Here's how the part is built. I have some questions about the finished solid (model axes, mm). A direction names the side the tool comes from. Round coordinates to 2 decimals unless told otherwise and drop trailing zeros. Loops run counter-clockwise (first coordinate to the right, second up) from the corner with the lowest first, then second, coordinate; pieces in that order, holes last. Notation, with made-up numbers: (33, 4.5) -> (90, 4.5) arc R15 ccw to (90, 22.5) -> close; hole circle Ø6 at (44.25, 57). An arc over 180 degrees is marked (long way). Use one line per item in the form item = value. Start each with the question number.
Item 1: If we section it at C-C (x = 0.5): Write out the boundary of the cut face in (y, z) (3 decimals), then the cut area to 3 significant figures.
Item 2: If I drill on L1, parallel to Z at x = -20, y = 0.85 (3 decimals); L2, parallel to X at y = 0.2, z = 5; L3, parallel to Z at x = 27.5, y = 0.6, over which ranges is the centre line in solid material (lowest first)? Write a range as [from, to].
Item 3: I'm going to push flat-ended pins straight in: pin 1 Ø1.6 at (x, y) = (2.5, 1.5) entering from -Z; pin 2 Ø2.5 at (x, z) = (20, 4.76) entering from -Y; pin 3 Ø1.5 at (y, z) = (0.5, 13) entering from -X; pin 4 Ø1.5 at (x, y) = (25.5, 2.5) entering from -Z. Where does each tip first touch, or does it pass through?
Item 4: If we section it at A-A (z = 13.75): Write out the boundary of the cut face in (x, y) (3 decimals), then the cut area to 3 significant figures.
Item 5: If we section it at B-B (y = 2.2): State how many separate pieces and enclosed holes the cut face has, then the cut area to 3 significant figures.
Item 6: For faces 5 (the face through (28.26, 1.61, 0.09)), 6 (the face through (14.097, 1.61, -0.154)), 7 (the face through (26.891, 1.61, -1.808)), 8 (the face through (21.4, 1.61, 14.14)), which set-ups out of +Z, -Z, +X, -X, +Y, -Y let a thin tool reach every point of the face, with its end or its side?
Item 7: Thinking about a two-plate mould opening in Z: for faces 1 (the face through (21.55, 1.61, -4.63)), 2 (the face through (25.12, 1.57, 10.53)), 3 (the face through (29.404, 1.61, 6.003)), 4 (the face through (26.903, 1.565, 8.178)), which applies, released by +Z, released by -Z, zero draft, split by the parting line, or undercut?
```python
from build123d import *

# Parameters (mm, degrees)
CROQUIS1_R              = 1.5875
SALIENTE_EXTRUIR1_DEPTH = 3.175
CROQUIS2_R              = 7.5
CROQUIS2_R_2            = 1.5875
SALIENTE_EXTRUIR2_DEPTH = 3.175
SALIENTE_EXTRUIR3_DEPTH = 3.175
CORTAR_EXTRUIR1_DEPTH   = 10
REDONDEO3_R             = 1
MATRIZC2_COUNT          = 7
MATRIZC2_ANGLE          = 222
REDONDEO3_OF_MATRIZC2_R = 1
REDONDEO4_R             = 2


with BuildPart() as part:
    # Croquis1 → Saliente-Extruir1 (new body)
    with BuildSketch(Plane(origin=(0, 0, 0), x_dir=(1, 0, 0), z_dir=(0, 1, 0))):
        with BuildLine():
            Line((-20, 0), (20, 0))
            ThreePointArc((20, 0), (24.7625, -4.7625), (20, -9.525))
            Line((20, -9.525), (-20, -9.525))
            ThreePointArc((-20, -9.525), (-24.7625, -4.7625), (-20, 0))
        make_face()
        with Locations((-20, -4.7625)):
            Circle(CROQUIS1_R, mode=Mode.SUBTRACT)
        with Locations((20, -4.7625)):
            Circle(CROQUIS1_R, mode=Mode.SUBTRACT)
    extrude(amount=SALIENTE_EXTRUIR1_DEPTH)

    # Croquis2 → Saliente-Extruir2 (add)
    with BuildSketch(Plane(origin=(0, 3.175, 0), x_dir=(1, 0, 0), z_dir=(0, 1, 0))):
        with Locations((20, -4.7625)):
            Circle(CROQUIS2_R)
        with Locations((20, -4.7625)):
            Circle(CROQUIS2_R_2, mode=Mode.SUBTRACT)
    extrude(amount=-SALIENTE_EXTRUIR2_DEPTH)

    # Croquis8 → Saliente-Extruir3 (add)
    with BuildSketch(Plane(origin=(0, 3.175, 0), x_dir=(1, 0, 0), z_dir=(0, 1, 0))):
        with BuildLine():
            Line((14.926688775, 5.835802374), (16.184441281, 1.694396442))
            ThreePointArc((16.184441281, 1.694396442), (17.363636492, 2.258866495), (18.622936274, 2.60999588))
            Line((18.622936274, 2.60999588), (16.844139666, 6.555761596))
            ThreePointArc((16.844139666, 6.555761596), (15.869697171, 6.237640842), (14.926688775, 5.835802374))
        make_face()
    saliente_extruir3 = extrude(amount=-SALIENTE_EXTRUIR3_DEPTH)

    # Croquis9 → Cortar-Extruir1 (cut)
    with BuildSketch(Plane(origin=(0, 3.175, 0), x_dir=(1, 0, 0), z_dir=(0, 1, 0))):
        with BuildLine():
            ThreePointArc((16.844139666, 6.555761596), (16.353447772, 6.407332445), (15.869697296, 6.237640889))
            ThreePointArc((15.869697296, 6.237640889), (16.670669085, 6.223682337), (17.245417982, 5.665637219))
            Line((17.245417982, 5.665637219), (16.844139666, 6.555761596))
        make_face()
        with BuildLine():
            ThreePointArc((15.869697296, 6.237640889), (15.393808961, 6.047009892), (14.926688775, 5.835802374))
            Line((14.926688775, 5.835802374), (15.210424872, 4.901543567))
            ThreePointArc((15.210424872, 4.901543567), (15.275853116, 5.699960746), (15.869697296, 6.237640889))
        make_face()
    cortar_extruir1 = extrude(amount=-CORTAR_EXTRUIR1_DEPTH, mode=Mode.SUBTRACT)

    # Redondeo3
    redondeo3_edges = [part.edges().sort_by_distance(p)[0] for p in [
        (18.622936274, 1.5875, -2.60999588),
        (16.184441281, 1.5875, -1.694396442),
    ]]
    fillet(redondeo3_edges, radius=REDONDEO3_R)

    # MatrizC2: Saliente-Extruir3, Cortar-Extruir1 ×7 about axis
    matrizc2_axis = Axis((20, 0, 4.7625), (0, -1, 0))
    for i in range(1, MATRIZC2_COUNT):
        add(saliente_extruir3.rotate(matrizc2_axis, i * MATRIZC2_ANGLE / (MATRIZC2_COUNT - 1)))
        add(cortar_extruir1.rotate(matrizc2_axis, i * MATRIZC2_ANGLE / (MATRIZC2_COUNT - 1)), mode=Mode.SUBTRACT)

    # Redondeo3 of MatrizC2
    redondeo3_of_matrizc2_edges = [part.edges().sort_by_distance(p)[0] for p in [
        (23.337106788, 1.5875, -1.954174645),
        (20.838616598, 1.5875, -2.690467342),
        (26.707327688, 1.5875, 1.406646118),
        (25.155056708, 1.5875, -0.685012307),
        (27.376313351, 1.5875, 6.118966491),
        (27.395406089, 1.5875, 3.514313802),
        (25.074643863, 1.5875, 10.284998498),
        (26.657411119, 1.5875, 8.216320666),
        (20.729268228, 1.5875, 12.226960319),
        (23.238283761, 1.5875, 11.527373856),
        (16.090195144, 1.5875, 11.16276765),
        (18.515005687, 1.5875, 12.114016299),
    ]]
    fillet(redondeo3_of_matrizc2_edges, radius=REDONDEO3_OF_MATRIZC2_R)

    # Redondeo4
    redondeo4_edges = [part.edges().sort_by_distance(p)[0] for p in [
        (14.206158981, 1.5875, 0),
        (14.206158981, 1.5875, 9.525),
    ]]
    fillet(redondeo4_edges, radius=REDONDEO4_R)


solid = part.part
```
Values found:
q1.outline = (0, 0) -> (3.175, 0) -> (3.175, 9.525) -> (0, 9.525) -> close
q1.area = 30.2 mm2
q2.L1 = [0, 3.175], [6.35, 9.525]
q2.L2 = [-24.76, -21.57], [-18.43, 18.43], [21.57, 31.74]
q2.L3 = [-2.2, 0.74], [3.27, 6.34], [8.95, 11.9]
q3.pin_1 = 0
q3.pin_2 = through
q3.pin_3 = 15.26
q3.pin_4 = -1.39
q4.outline = (15.263, 0) -> (17.748, 0) -> (17.748, 3.175) -> (15.263, 3.175) -> close; (21.262, 0) -> (23.706, 0) -> (23.706, 3.175) -> (21.262, 3.175) -> close
q4.area = 15.7 mm2
q5.separate_pieces = 1
q5.enclosed_holes = 2
q5.area = 579 mm2
q6.face_5 = +X, +Y, -Y
q6.face_6 = -Z, -X, +Y, -Y
q6.face_7 = -Z, +Y, -Y
q6.face_8 = +Z, +Y, -Y
q7.face_1 = released by -Z
q7.face_2 = released by +Z
q7.face_3 = undercut
q7.face_4 = undercut
